Geometry: final body of the model. Coordinates: model frame, mm. Coordinates: 2 decimals unless noted, no trailing zeros. Order: outer loops, then holes, each group sorted by start corner. A loop starts at its lowest first (then second) coordinate and runs counter-clockwise, first axis right, second up. Notation, with made-up numbers: (81.5, 88) - (126.5, 88) arc R29 cw to (126.5, 108) - close; hole circle Ø5 at (69.5, -7). An arc over 180 degrees is marked (long way). Use a Markdown table: item, result. Add a question column.
```python
from build123d import *

# Parameters (mm, degrees)
SKETCH1_W           = 81
SKETCH1_H           = 153
BOSS_EXTRUDE1_DEPTH = 3
CUT_EXTRUDE2_DEPTH  = 81
CUT_EXTRUDE3_DEPTH  = 81
SKETCH6_W           = 1.85
SKETCH6_H           = 1.55
CUT_EXTRUDE5_DEPTH  = 0.6
FILLET6_R           = 0.4
CHAMFER2_SIZE       = 0.2
SKETCH7_W           = 1.85
SKETCH7_H           = 1.55
CUT_EXTRUDE6_DEPTH  = 0.6
FILLET7_R           = 0.4
CHAMFER3_SIZE       = 0.2
SKETCH10_W          = 81
SKETCH10_H          = 150.1
CUT_EXTRUDE7_DEPTH  = 0.2
FILLET8_R           = 0.4
BOSS_EXTRUDE2_DEPTH = 3
FILLET10_R          = 0.5


with BuildPart() as part:
    # Sketch1 → Boss-Extrude1 (new body)
    with BuildSketch(Plane(origin=(0, 0, 0), x_dir=(1, 0, 0), z_dir=(0, 1, 0))):
        with Locations((40.5, 76.5)):
            Rectangle(SKETCH1_W, SKETCH1_H)
    extrude(amount=BOSS_EXTRUDE1_DEPTH)

    # Sketch2 → Cut-Extrude2 (cut)
    with BuildSketch(Plane(origin=(81, 0, 0), x_dir=(0, 0, -1), z_dir=(1, 0, 0))):
        Polygon((0, 3), (3, 3), (3, 1.75), (1.25, 1.75), (1.25, 0), (0, 0), align=None)
        Polygon((151.75, 0), (153, 0), (153, 3), (150, 3), (150, 1.75), (151.75, 1.75), align=None)
    extrude(amount=-CUT_EXTRUDE2_DEPTH, mode=Mode.SUBTRACT)

    # Sketch4 → Cut-Extrude3 (cut)
    with BuildSketch(Plane(origin=(81, 0, 0), x_dir=(0, 0, -1), z_dir=(1, 0, 0))):
        Polygon((3.2, 3), (3, 3), (3, 1.75), (1.25, 1.75), (1.25, 0), (1.45, 0), (1.45, 1.55), (3.2, 1.55), align=None)
        Polygon((151.75, 0), (151.55, 0), (151.55, 1.55), (149.8, 1.55), (149.8, 3), (150, 3), (150, 1.75), (151.75, 1.75), align=None)
    extrude(amount=-CUT_EXTRUDE3_DEPTH, mode=Mode.SUBTRACT)

    # Sketch6 → Cut-Extrude5 (cut)
    with BuildSketch(Plane.XY.offset(-1.45)):
        with Locations((3, 0.775)):
            Rectangle(SKETCH6_W, SKETCH6_H)
    extrude(amount=-CUT_EXTRUDE5_DEPTH, mode=Mode.SUBTRACT)

    # Fillet6
    fillet6_edges = [part.edges().sort_by_distance(p)[0] for p in [
        (2.075, 0.775, -1.45),
    ]]
    fillet(fillet6_edges, radius=FILLET6_R)

    # Chamfer2
    chamfer2_edges = [part.edges().sort_by_distance(p)[0] for p in [
        (3.925, 0.775, -1.45),
    ]]
    chamfer(chamfer2_edges, length=CHAMFER2_SIZE)

    # Sketch7 → Cut-Extrude6 (cut)
    with BuildSketch(Plane(origin=(0, 0, -151.55), x_dir=(-1, 0, 0), z_dir=(0, 0, -1))):
        with Locations((-3, 0.775)):
            Rectangle(SKETCH7_W, SKETCH7_H)
    extrude(amount=-CUT_EXTRUDE6_DEPTH, mode=Mode.SUBTRACT)

    # Fillet7
    fillet7_edges = [part.edges().sort_by_distance(p)[0] for p in [
        (2.075, 0.775, -151.55),
    ]]
    fillet(fillet7_edges, radius=FILLET7_R)

    # Chamfer3
    chamfer3_edges = [part.edges().sort_by_distance(p)[0] for p in [
        (3.925, 0.775, -151.55),
    ]]
    chamfer(chamfer3_edges, length=CHAMFER3_SIZE)

    # Sketch10 → Cut-Extrude7 (cut)
    with BuildSketch(Plane(origin=(0, 0, 0), x_dir=(-1, 0, 0), z_dir=(0, -1, 0))):
        with Locations((-40.5, 76.5)):
            Rectangle(SKETCH10_W, SKETCH10_H)
    extrude(amount=-CUT_EXTRUDE7_DEPTH, mode=Mode.SUBTRACT)

    # Fillet8
    fillet8_edges = [part.edges().sort_by_distance(p)[0] for p in [
        (0, 0.875, -151.55),
        (0, 0.875, -1.45),
    ]]
    fillet(fillet8_edges, radius=FILLET8_R)

    # Sketch9 → Boss-Extrude2 (add)
    with BuildSketch(Plane(origin=(0, 3, 0), x_dir=(1, 0, 0), z_dir=(0, 1, 0))):
        with BuildLine():
            Line((74.5, 43), (74.5, 110))
            ThreePointArc((74.5, 110), (76, 111.5), (77.5, 110))
            Line((77.5, 110), (77.5, 43))
            ThreePointArc((77.5, 43), (76, 41.5), (74.5, 43))
        make_face()
    extrude(amount=BOSS_EXTRUDE2_DEPTH)

    # Fillet10
    fillet10_edges = [part.edges().sort_by_distance(p)[0] for p in [
        (76, 3, -41.5),
        (77.5, 3, -76.5),
        (76, 3, -111.5),
        (74.5, 3, -76.5),
        (76, 6, -41.5),
        (77.5, 6, -76.5),
        (76, 6, -111.5),
        (74.5, 6, -76.5),
    ]]
    fillet(fillet10_edges, radius=FILLET10_R)


solid = part.part
```
1) Section B-B (z = -115.5). Return loops of the section in (x, y), then the cut area to 3 significant figures.
2) Section A-A (x = 61.5). Return loops of the section in (y, z).
3) Pin query (flat end, axial travel): pin 1 (1.5 mm diameter, centred on y = 3, z = -92.5, fed in from -X); pin 2 (3 mm diameter, centred on x = 65, y = 3.5, fed in from -Z); pin 3 (0.9 mm diameter, centred on x = 51, z = -150.5, fed in from +Y); pin 4 (1 mm diameter, centred on y = 5, z = -74, fed in from -X). Return the tip coordinate at first contact, or that it passes through.
4) Ray query, line 1 along Y through (x, z) = (37, -27); line 2 along X through (y, z) = (5.35, -46); line 3 along Z through (x, y) = (48.5, 1.9). Return the intervals inside material, ascending.
Values follow:
| question | item | result |
|---|---|---|
| 1 | outline | (0, 0.2) - (81, 0.2) - (81, 3) - (0, 3) - close |
| 1 | area | 227 mm² |
| 2 | outline | (0.2, -151.55) - (1.55, -151.55) - (1.55, -149.8) - (3, -149.8) - (3, -3.2) - (1.55, -3.2) - (1.55, -1.45) - (0.2, -1.45) - close |
| 3 | pin 1 | stops at x = 0 |
| 3 | pin 2 | stops at z = -149.8 |
| 3 | pin 3 | stops at y = 1.55 |
| 3 | pin 4 | stops at x = 74.5 |
| 4 | line 1 | y = 0.2 to 3 |
| 4 | line 2 | x = 74.5 to 77.5 |
| 4 | line 3 | z = -149.8 to -3.2 |
